Input: dimensioned drawing with shaded views. Units: mm. Origin: part minimum x, y, z. A direction names the side the tool comes from. Give positions to 0.01 mm unless a question says otherwise; leave off trailing zeros. Write each loop counter-clockwise with the first axis right and the second up, starting at its lowest first coordinate (ties: lowest second). Pieces come first, ordered by that corner, then holes. Notation, with made-up numbers: (-27, 28.25) -> (32, 28.25) arc R23 cw to (32, 41.25) -> close; hole circle Ø9 at (37, 16.5). An arc over 180 degrees is marked (long way). Return JSON: item names as keys, results as strings. Group by question number.
Item 1: Pin query (flat end, axial travel): P1, Ø5, axis at x = 13.5, y = 17.5, coming from the -Z side. Return the tip coordinate at first contact, or that it passes through.
Item 2: Section A-A, the plane x = 18.5. Return loops of the section in (y, z).
Item 3: Section D-D, the plane y = 3.75. Return loops of the section in (x, z), then the cut area to 3 significant figures.
Item 4: Section C-C, the plane y = 12. Return loops of the section in (x, z).
Item 5: Set-up query: the marked faces 5 and 6. Return all of +Z, -Z, +X, -X, +Y, -Y with unobstructed straight access to the full face (end or side cutting, diameter ignored); none if empty.
Item 6: Line query: line 1 (Y direction, x = 9, z = 4.5); line 2 (Z direction, x = 13, y = 3.5). Output: solid intervals per line, ascending. Write a range as [from, to].
Item 7: Mould query, pull axis Y, two halves, no side actions, for the marked faces 1, 2, 3 and 4. Classes: released by +Y, released by -Y, zero draft, split by the parting line, or undercut.
Item 8: Section B-B, the plane z = 4. Return loops of the section in (x, y).
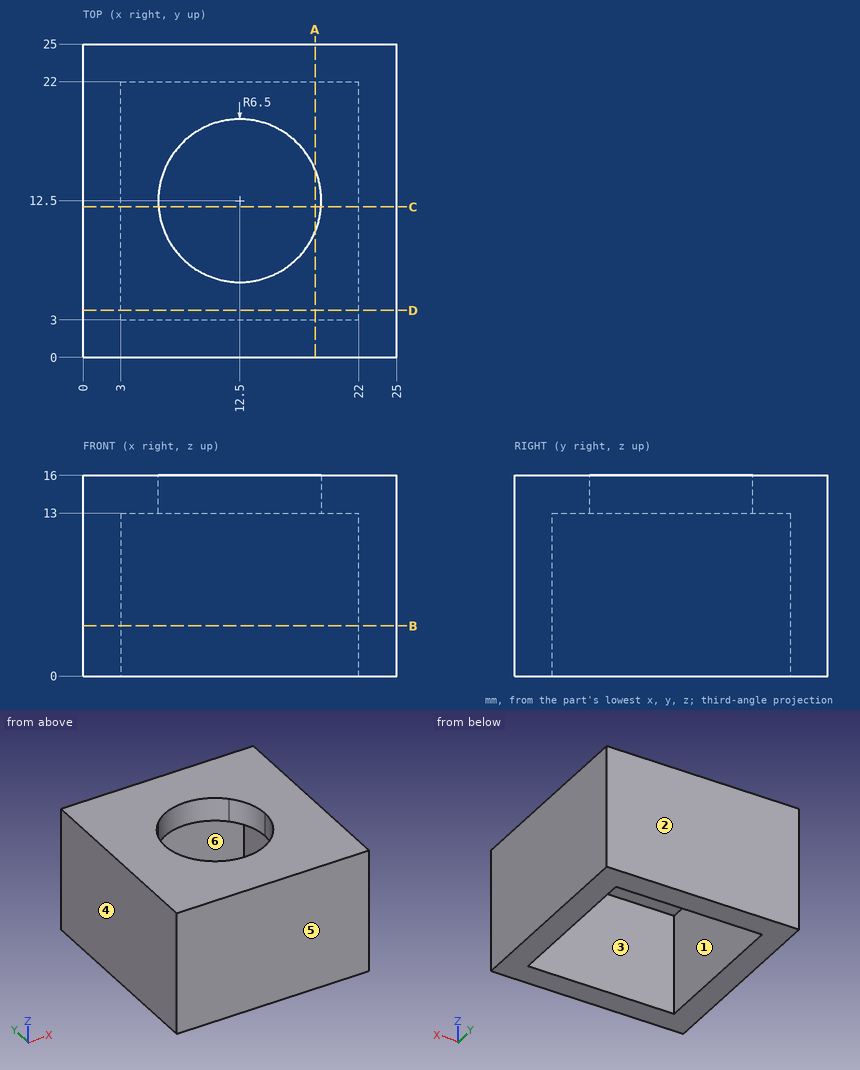
Answer below:
{
 "1": {"P1": "stops at z = 13"},
 "2": {"outline": "(0, 0) -> (3, 0) -> (3, 13) -> (10, 13) -> (10, 16) -> (0, 16) -> close; (15, 13) -> (22, 13) -> (22, 0) -> (25, 0) -> (25, 16) -> (15, 16) -> close"},
 "3": {"outline": "(0, 0) -> (3, 0) -> (3, 13) -> (22, 13) -> (22, 0) -> (25, 0) -> (25, 16) -> (0, 16) -> close", "area": "153 mm2"},
 "4": {"outline": "(0, 0) -> (3, 0) -> (3, 13) -> (6.02, 13) -> (6.02, 16) -> (0, 16) -> close; (18.98, 13) -> (22, 13) -> (22, 0) -> (25, 0) -> (25, 16) -> (18.98, 16) -> close"},
 "5": {"face 5": "+Z, -Z, +X, -X, -Y", "face 6": "-Z"},
 "6": {"line 1": "y = [0, 3], [22, 25]", "line 2": "z = [13, 16]"},
 "7": {"face 1": "undercut", "face 2": "released by +Y", "face 3": "undercut", "face 4": "zero draft"},
 "8": {"outline": "(0, 0) -> (25, 0) -> (25, 25) -> (0, 25) -> close; hole (3, 3) -> (22, 3) -> (22, 22) -> (3, 22) -> close"}
}
